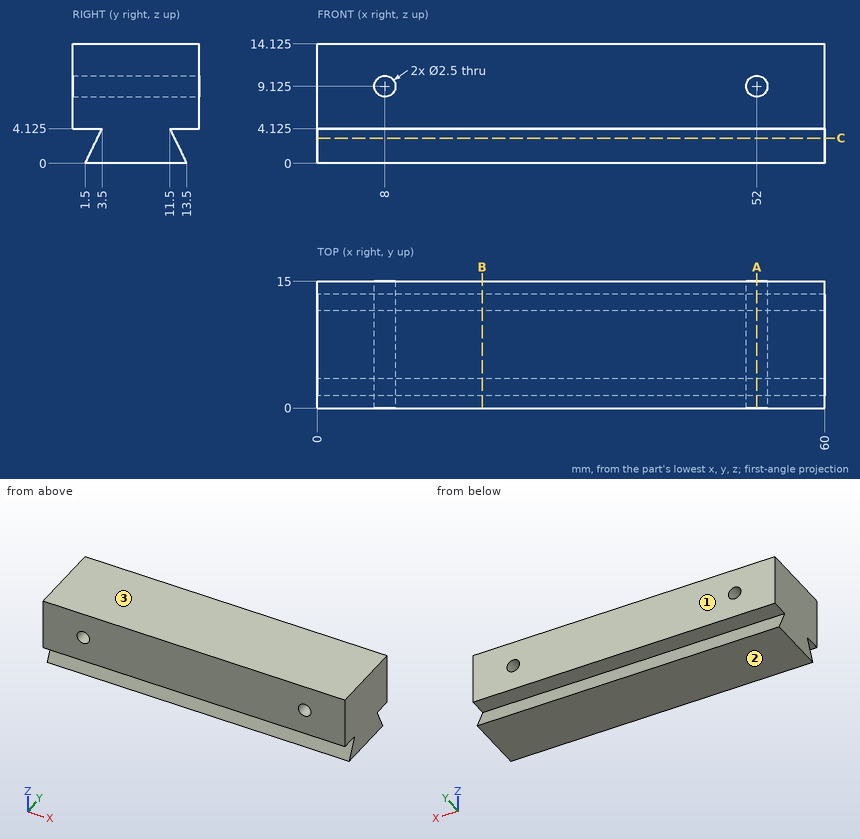
For this review, use the dimensioned drawing (mm, ordinates from the lowest corner) and the shaded views. Round coordinates to 2 decimals unless told otherwise and drop trailing zeros. Order: outer loops, then holes, each group sorted by start corner. A loop starts at its lowest first (then second) coordinate and runs counter-clockwise, first axis right, second up.
1) Clearance check with a flat-ended pin moving along its axis: pin 1 Ø3 at (x, z) = (41.5, 2) entering from +Y. State where the tip first meets the part, or that it passes through.
The answers:
pin 1: stops at y = 13.26
2) Consider section A-A (x = 52). State the section outline as (y, z) points (1 decimal).
The answers:
outline: (0, 4.1) - (3.5, 4.1) - (1.5, 0) - (13.5, 0) - (11.5, 4.1) - (15, 4.1) - (15, 7.9) - (0, 7.9) - close; (0, 10.4) - (15, 10.4) - (15, 14.1) - (0, 14.1) - close
3) Draft analysis for pull direction Z (two halves, no side actions). For the marked faces 1, 2 and 3, state which applies: released by +Z, released by -Z, zero draft, split by the parting line, or undercut.
The answers:
face 1: zero draft
face 2: released by -Z
face 3: released by +Z
4) Consider section C-C (z = 3). State the section outline as (x, y) points, plus the area to 3 significant figures.
The answers:
outline: (0, 2.95) - (60, 2.95) - (60, 12.05) - (0, 12.05) - close
area: 545 mm2
5) Consider section B-B (x = 19.5). State the section outline as (y, z) points (1 decimal), plus the area to 3 significant figures.
The answers:
outline: (0, 4.1) - (3.5, 4.1) - (1.5, 0) - (13.5, 0) - (11.5, 4.1) - (15, 4.1) - (15, 14.1) - (0, 14.1) - close
area: 191 mm2
6) For L1, parallel to X at y = 2.75, z = 9.25; L2, parallel to Z at x = 8, y = 10.75 (1 decimal); L3, parallel to X at y = 4.5, z = 8 (1 decimal), list the stretches that pass through material, from the lowest coordinate up.
The answers:
L1: x = 0 to 6.76, 9.24 to 50.76, 53.24 to 60
L2: z = 0 to 7.9, 10.4 to 14.1
L3: x = 0 to 7.5, 8.5 to 51.5, 52.5 to 60
